Can you work these out from the model? Positions are in its coordinate system, mm. Face numbers are marked on the shaded views. A direction names the side the tool comes from. Give positions to 0.01 mm unless a question says otherwise; leave off trailing zeros. Loops run counter-clockwise (first coordinate to the right, second up) from the corner with the lowest first, then second, coordinate; pieces in that order, holes last. Notation, with made-up numbers: M 59.25,49.5 L 118.25,49.5 A20 cw 118.25,79.5 Z; hole C 72,-37 d4. An arc over 180 degrees is marked long. Answer as a JSON object with one key per item and string values.
```python
from build123d import *

# Parameters (mm, degrees)
F0_W     = 101.6
F0_H     = 50.8
F1_DEPTH = 76.2
F2_W     = 76.2
F2_H     = 25.4
F3_DEPTH = 50.8
F5_DEPTH = 25.4
F7_DEPTH = 25.4


with BuildPart() as f1:
    # F0 (on Front) → F1 (new body)
    with BuildSketch(Plane.XZ):
        with Locations((-24.98975, 25.4)):
            Rectangle(F0_W, F0_H)
    extrude(amount=F1_DEPTH)

    # F2 (on face) → F3 (join)
    with BuildSketch(Plane.YZ.offset(25.81025)):
        with Locations((-38.1, 12.7)):
            Rectangle(F2_W, F2_H)
    extrude(amount=F3_DEPTH)

    # F4 (on face) → F5 (cut)
    with BuildSketch(Plane.XY.offset(25.4)):
        Polygon((25.81025, -50.8), (25.81025, -76.2), (76.61025, -76.2), (76.61025, -74.655533), align=None)
    extrude(amount=-F5_DEPTH, mode=Mode.SUBTRACT)

    # F6 (on face) → F7 (cut)
    with BuildSketch(Plane.XY.offset(25.4)):
        Polygon((25.81025, 0), (25.81025, -25.4), (76.61025, 0), align=None)
    extrude(amount=-F7_DEPTH, mode=Mode.SUBTRACT)


solid = f1.part
```
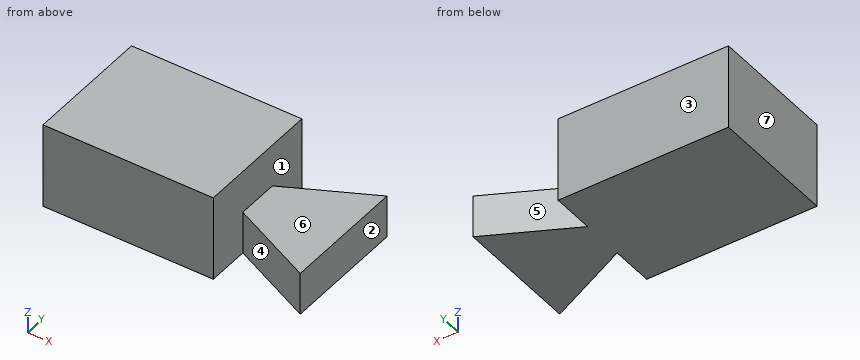
1) Suppose I cut it at C-C, the plane y = -27.5. Write out the boundary of the cut face in (x, z).
Answer list:
{"outline": "M -75.79,0 L 76.61,0 L 76.61,25.4 L 25.81,25.4 L 25.81,50.8 L -75.79,50.8 Z"}
2) Suppose I cut it at D-D, the plane x = 63. Write out the boundary of the cut face in (y, z).
Answer list:
{"outline": "M -68.26,0 L -6.81,0 L -6.81,25.4 L -68.26,25.4 Z"}
3) Will this pin go through, and if not, where does the flat tip stop? pin 1 Ø12 at (y, z) = (-37.5, 33) entering from +X.
Answer list:
{"pin 1": "x = 25.81"}
4) For the marked faces 5, 6 and 7, which set-ups out of +Z, -Z, +X, -X, +Y, -Y let a thin tool reach every point of the face, with its end or its side?
Answer list:
{"face 5": "+Z, -Z, +Y", "face 6": "+Z, +X, +Y, -Y", "face 7": "+Z, -Z, -X, +Y, -Y"}
5) Suppose I cut it at B-B, the plane z = 21.5. Write out the boundary of the cut face in (x, y), and give its area (3 significant figures).
Answer list:
{"outline": "M -75.79,-76.2 L 25.81,-76.2 L 25.81,-50.8 L 76.61,-74.66 L 76.61,0 L 25.81,-25.4 L 25.81,0 L -75.79,0 Z", "area": "10,300 mm^2"}
6) Please list where these lines run through material, in increasing order: line 1 along X through (y, z) = (-40, 36); line 2 along Z through (x, y) = (60, -19); line 3 along X through (y, z) = (-54.5, 6). Write a range as from..to.
Answer list:
{"line 1": "-75.79..25.81", "line 2": "0..25.4", "line 3": "-75.79..25.81, 33.69..76.61"}
7) Suppose I cut it at A-A, the plane y = -10.5. Write out the boundary of the cut face in (x, z).
Answer list:
{"outline": "M -75.79,0 L 25.81,0 L 25.81,50.8 L -75.79,50.8 Z; M 55.61,0 L 76.61,0 L 76.61,25.4 L 55.61,25.4 Z"}
8) If we mould it in two halves opening along X, with no side actions, what happens to the marked faces 1, 2, 3 and 4? For each: +X half, -X half, draft (parallel to the pull), parting line (faces both ways), or undercut.
Answer list:
{"face 1": "undercut", "face 2": "+X half", "face 3": "draft", "face 4": "undercut"}
